Can you work these out from the drawing? Everything is in mm from the part's minimum corner. A direction names the side the tool comes from. Give positions to 0.01 mm unless a question says otherwise; leave off trailing zeros. Order: outer loops, then holes, each group sorted by start corner. A loop starts at its lowest first (then second) coordinate and runs counter-clockwise, first axis right, second up. Notation, with made-up numbers: (33, -35) -> (71, -35) arc R36 ccw to (71, 1) -> close; hole circle Ø6 at (14.5, 80.25). An arc over 180 degrees is marked (long way). Answer as CSV lines item,"result". Start each with the question number.
(1) I need wall thicknesses on L1, parallel to Z at x = 97.75, y = 7.5; L2, parallel to X at y = 2, z = 42.5; L3, parallel to Y at x = 96.4, z = 7.5. Which ranges of each line are inside material? Lowest first, please.
(2) On a 3-axis mill with a long thin cutter (end or side, diameter ignored), from which of +Z, -Z, +X, -X, +Y, -Y can I reach the whole of each face in a straight line? I mean the marked faces 1 and 2. Say none if no direction works.
(3) I want a section at B-B (y = 7.5). Please give me the cut outline in (x, z).
(4) Will these pins go through, and if not, where does the flat tip stop? pin 1 Ø3 at (y, z) = (42.5, 7.5) entering from -X; pin 2 Ø4 at (x, z) = (13.5, 12) entering from +Y; pin 3 Ø1.6 at (x, y) = (32, 44.5) entering from +Z.
(5) I want a section at C-C (x = 21.5). Please give me the cut outline in (y, z).
(6) I want a section at A-A (z = 47.5). Please give me the cut outline in (x, y).
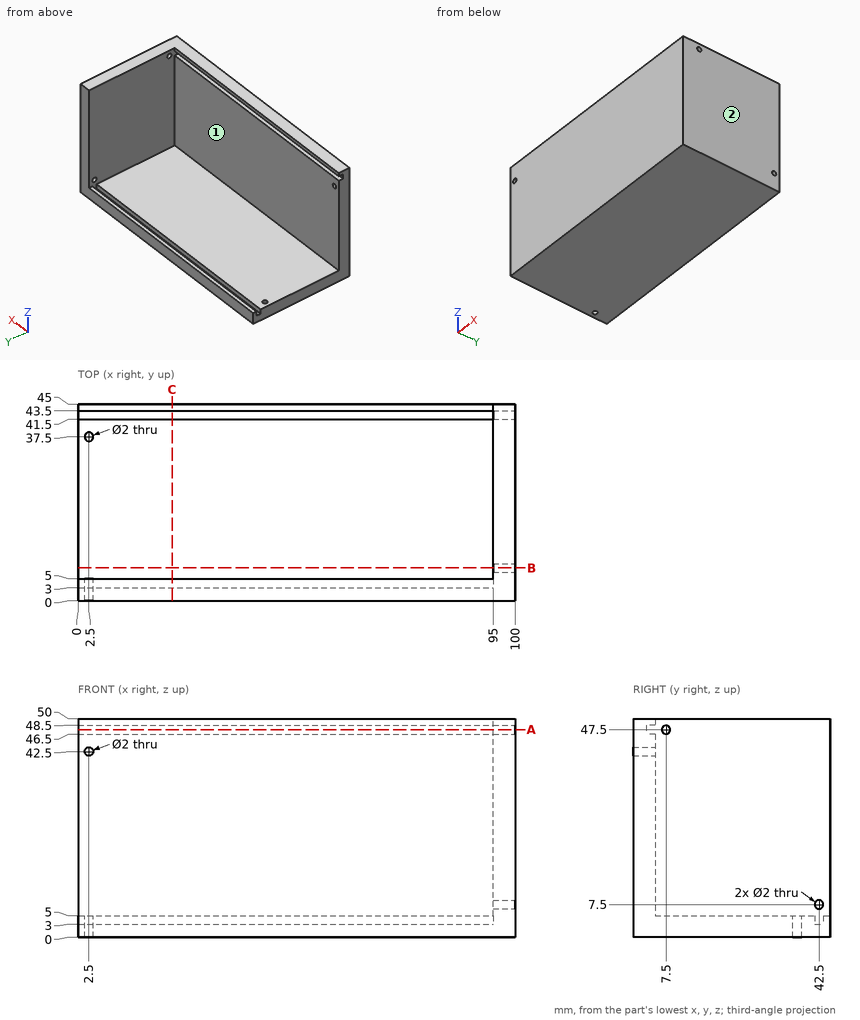
Final values:
1,L1,"0 to 46.5, 48.5 to 50"
1,L2,"0 to 1.5, 3.5 to 100"
1,L3,"0 to 41.5, 43.5 to 45"
2,face 1,"+Z, -X, +Y"
2,face 2,"+Z, -Z, +X, +Y, -Y"
3,outline,"(0, 0) -> (100, 0) -> (100, 46.5) -> (95, 46.5) -> (95, 5) -> (0, 5) -> close; (95, 48.5) -> (100, 48.5) -> (100, 50) -> (95, 50) -> close"
4,pin 1,"x = 95"
4,pin 2,"y = 5"
4,pin 3,"z = 5"
5,outline,"(0, 0) -> (45, 0) -> (45, 5) -> (43.5, 5) -> (43.5, 3) -> (41.5, 3) -> (41.5, 5) -> (5, 5) -> (5, 46.5) -> (3, 46.5) -> (3, 48.5) -> (5, 48.5) -> (5, 50) -> (0, 50) -> close"
6,outline,"(0, 0) -> (100, 0) -> (100, 6.5) -> (95, 6.5) -> (95, 3) -> (0, 3) -> close; (95, 8.5) -> (100, 8.5) -> (100, 45) -> (95, 45) -> close"
